```python
from build123d import *

# Parameters (mm, degrees)
SKETCH1_W                = 38.1
SKETCH1_H                = 203.2
BOSS_EXTRUDE1_DEPTH      = 7.9375
O_0_316_DIAMETER_HOLE1_D = 8.0264
SKETCH4_R                = 8.89
BOSS_EXTRUDE2_DEPTH      = 12.7


with BuildPart() as part:
    # Sketch1 → Boss-Extrude1 (new body)
    with BuildSketch(Plane.XY):
        Rectangle(SKETCH1_W, SKETCH1_H)
    extrude(amount=BOSS_EXTRUDE1_DEPTH)

    # O (0.316) Diameter Hole1 (through all)
    with Locations(Plane.XY.offset(7.9375)):
        with Locations((0, 88.9)):
            o_0_316_diameter_hole1 = Hole(O_0_316_DIAMETER_HOLE1_D / 2)

    # Mirror1: O (0.316) Diameter Hole1 across plane
    add(o_0_316_diameter_hole1.mirror(Plane.ZX), mode=Mode.SUBTRACT)

    # Sketch4 → Boss-Extrude2 (add)
    with BuildSketch(Plane.XY.offset(7.9375)):
        with Locations((-9.144, 63.5)):
            Circle(SKETCH4_R)
        with Locations((9.144, 63.5)):
            Circle(SKETCH4_R)
    extrude(amount=BOSS_EXTRUDE2_DEPTH)


solid = part.part
```
CAD build for the part. Positions are in the model's coordinates, mm. A direction names the side the tool comes from. Coordinates: 2 decimals unless noted, no trailing zeros. Loops run counter-clockwise (first coordinate to the right, second up) from the corner with the lowest first, then second, coordinate; pieces in that order, holes last. Notation, with made-up numbers: (0, 84.5) - (50, 84.5) arc R26 cw to (50, 108.5) - close; hole circle Ø6 at (-12.5, 43.5). An arc over 180 degrees is marked (long way). Return JSON: item names as keys, results as strings.
1. 3-axis set-ups, long thin cutter, end or side, ignore diameter. For faces 4 (the cylindrical face through (0.52, -92.88, 3.91)), 5 (the cylindrical face through (13.246, 55.613, 14.199)): which of +Z, -Z, +X, -X, +Y, -Y reach the whole face in a straight line?
Result:
{"face 4": "+Z, -Z", "face 5": "+Z"}
2. Band-saw the part on C-C (x = 2). Give the cut face in (y, z), and give its area (3 significant figures).
Result:
{"outline": "(-101.6, 0) - (-92.38, 0) - (-92.38, 7.94) - (-101.6, 7.94) - close; (-85.42, 0) - (85.42, 0) - (85.42, 7.94) - (68.79, 7.94) - (68.79, 20.64) - (58.21, 20.64) - (58.21, 7.94) - (-85.42, 7.94) - close; (92.38, 0) - (101.6, 0) - (101.6, 7.94) - (92.38, 7.94) - close", "area": "1,640 mm2"}
3. Mould opens along X. For faces 1 (the cylindrical face through (0.52, 92.88, 3.91)), 2 (the flat face through (-9, 64, 20.638)), 3 (the flat face through (19.05, -1, 4)) say: released by +X, released by -X, zero draft, split by the parting line, or undercut.
Result:
{"face 1": "undercut", "face 2": "zero draft", "face 3": "released by +X"}
4. Band-saw the part on B-B (z = 12.25). Give the cut face in (x, y), and give its area (3 significant figures).
Result:
{"outline": "circle Ø17.78 at (-9.14, 63.5); circle Ø17.78 at (9.14, 63.5)", "area": "497 mm2"}
5. Probe L1, parallel to Y at x = 0, z = 2.75; L2, parallel to Z at x = -11, y = 49.5; L3, parallel to Y at x = -3, z = 19. List the from-to ranges inside material, lowest first. Write a range as from..to.
Result:
{"L1": "y = -101.6..-92.91, -84.89..84.89, 92.91..101.6", "L2": "z = 0..7.94", "L3": "y = 57.07..69.93"}
6. Band-saw the part on D-D (y = 63.5). Give the cut face in (x, z).
Result:
{"outline": "(-19.05, 0) - (19.05, 0) - (19.05, 7.94) - (18.03, 7.94) - (18.03, 20.64) - (0.25, 20.64) - (0.25, 7.94) - (-0.25, 7.94) - (-0.25, 20.64) - (-18.03, 20.64) - (-18.03, 7.94) - (-19.05, 7.94) - close"}
7. Band-saw the part on A-A (y = 88.9). Give the cut face in (x, z), and give its area (3 significant figures).
Result:
{"outline": "(-19.05, 0) - (-4.01, 0) - (-4.01, 7.94) - (-19.05, 7.94) - close; (4.01, 0) - (19.05, 0) - (19.05, 7.94) - (4.01, 7.94) - close", "area": "239 mm2"}
8. Drop flat-ended pins along their axis: pin 1 (1.5 mm diameter, centred on x = -6, y = -24.5, fed in from +Z); pin 2 (2 mm diameter, centred on x = 7, z = 11.5, fed in from +Y). Give the stop position or say it passes through.
Result:
{"pin 1": "stops at z = 7.94", "pin 2": "stops at y = 72.32"}
